Study the drawing (mm; zero at the part's minimum x, y, z) and answer. Round coordinates to 2 decimals unless told otherwise and drop trailing zeros. Loops run counter-clockwise (first coordinate to the right, second up) from the corner with the lowest first, then second, coordinate; pieces in that order, holes last. Notation, with made-up numbers: M 43.25,52 L 53.25,52 A29 ccw 53.25,88 Z; hole C 20,44.25 d2. An arc over 180 degrees is marked long. Put each result on its own line as item: value. Start each with the question number.
(1) Straight lines are drawn through the part: line 1 (X direction, y = 4.75, z = 12.7) (1 decimal); line 2 (X direction, y = 4, z = 4.5); line 3 (X direction, y = 5, z = 3.75). For each, find the intervals that lie inside material, in ascending order.
(2) Section B-B, the plane x = 57.15 is taken. Count the separate pieces of the cut face and the enclosed holes in it, then the cut area to 3 significant figures.
(3) Section A-A, the plane x = 25.4 is taken. Determine the outline of the cut face in (y, z), then the cut area to 3 significant figures.
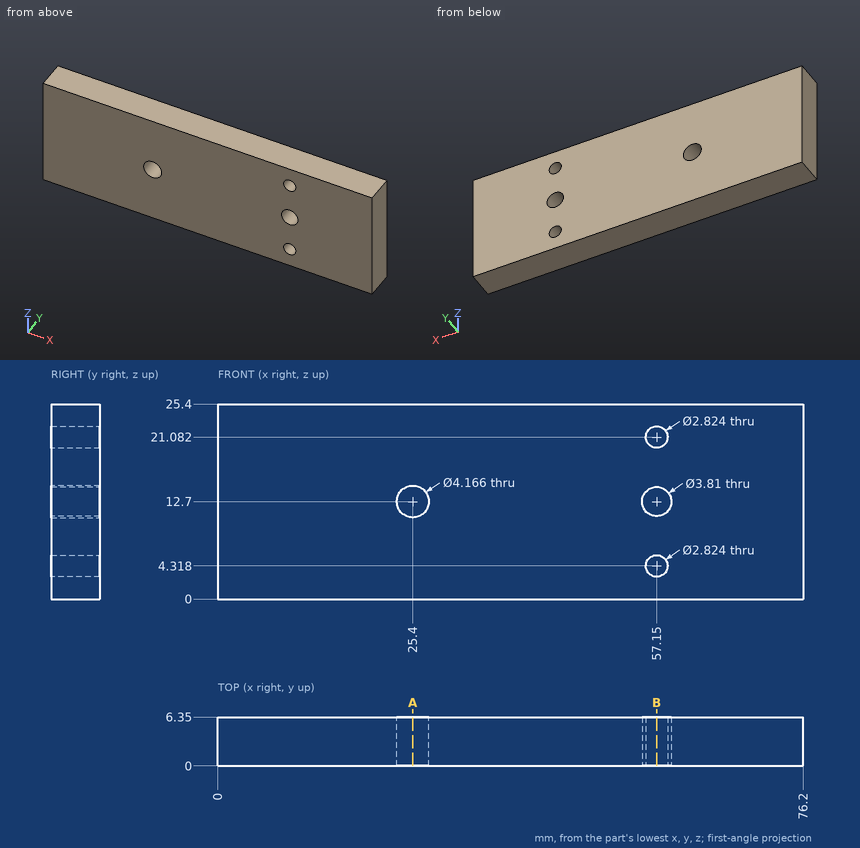
Recorded:
1. line 1: x = 0 to 23.3, 27.5 to 55.2, 59.1 to 76.2
1. line 2: x = 0 to 55.75, 58.55 to 76.2
1. line 3: x = 0 to 55.86, 58.44 to 76.2
2. separate pieces: 4
2. enclosed holes: 0
2. area: 101 mm²
3. outline: M 0,0 L 6.35,0 L 6.35,10.62 L 0,10.62 Z; M 0,14.78 L 6.35,14.78 L 6.35,25.4 L 0,25.4 Z
3. area: 135 mm²
